Could you check a few things on this drawing? It's one solid part, dimensions in mm from its lowest x, y, z. Give positions to 0.01 mm unless a question says otherwise; leave off trailing zeros. Order: outer loops, then holes, each group sorted by start corner. A loop starts at its lowest first (then second) coordinate and runs counter-clockwise, first axis right, second up. Notation, with made-up numbers: (5, 46) - (63, 46) arc R17 cw to (63, 74) - close; hole circle Ø7 at (35.5, -39). An arc over 180 degrees is marked (long way). Answer as CSV lines item,"result".
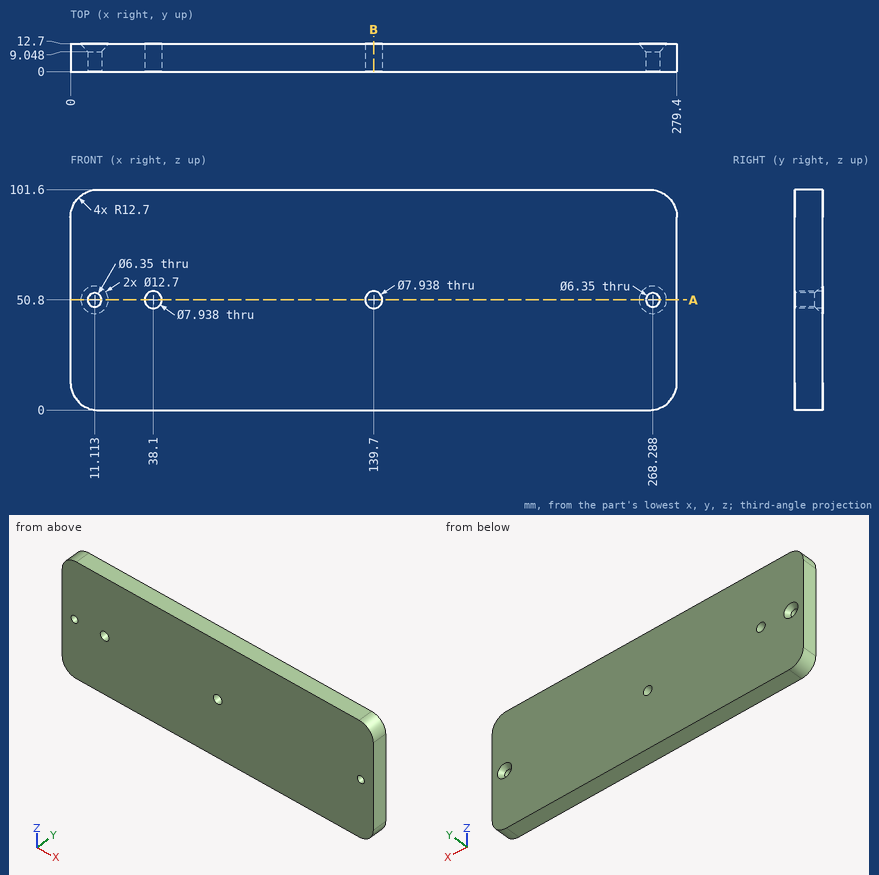
1) I want a section at A-A on z = 50.8. Write out the boundary of the cut face in (x, y), plus the area to 3 significant figures.
Answer block:
outline,"(0, 0) - (7.94, 0) - (7.94, 9.05) - (4.76, 12.7) - (0, 12.7) - close; (14.29, 0) - (34.13, 0) - (34.13, 12.7) - (17.46, 12.7) - (14.29, 9.05) - close; (42.07, 0) - (135.73, 0) - (135.73, 12.7) - (42.07, 12.7) - close; (143.67, 0) - (265.11, 0) - (265.11, 9.05) - (261.94, 12.7) - (143.67, 12.7) - close; (271.46, 0) - (279.4, 0) - (279.4, 12.7) - (274.64, 12.7) - (271.46, 9.05) - close"
area,"3,160 mm2"
2) I need wall thicknesses on line 1 along Z through (x, y) = (139.7, 4); line 2 along X through (y, z) = (1, 53.5) (1 decimal); line 3 along X through (y, z) = (1.5, 52). Which ranges of each line are inside material? Lowest first, please. Write a range as [from, to].
Answer block:
line 1,"[0, 46.83], [54.77, 101.6]"
line 2,"[0, 9.4], [12.8, 35.2], [41, 136.8], [142.6, 266.6], [270, 279.4]"
line 3,"[0, 8.17], [14.05, 34.32], [41.88, 135.92], [143.48, 265.35], [271.23, 279.4]"
3) I want a section at B-B on x = 139.7. Write out the boundary of the cut face in (y, z), plus the area to 3 significant figures.
Answer block:
outline,"(0, 0) - (12.7, 0) - (12.7, 46.83) - (0, 46.83) - close; (0, 54.77) - (12.7, 54.77) - (12.7, 101.6) - (0, 101.6) - close"
area,"1,190 mm2"
